Could you check a few things on this model? Use its own coordinates, in mm. A direction names the side the tool comes from. Give positions to 0.01 mm unless a question says otherwise; leave off trailing zeros. Order: outer loops, then holes, each group sorted by start corner. A loop starts at its lowest first (then second) coordinate and runs counter-clockwise, first axis right, second up.
from build123d import *

# Parameters (mm, degrees)
CROQUIS1_W              = 35
CROQUIS1_H              = 28
CROQUIS1_R              = 11
CROQUIS1_R_2            = 1.5
SALIENTE_EXTRUIR1_DEPTH = 10
CROQUIS2_R              = 11
CROQUIS2_R_2            = 9
SALIENTE_EXTRUIR2_DEPTH = 2
REDONDEO1_R             = 14
CHAFL_N1_SIZE           = 2


with BuildPart() as part:
    # Croquis1 → Saliente-Extruir1 (new body)
    with BuildSketch(Plane(origin=(0, 0, 0), x_dir=(0, 1, 0), z_dir=(0, 0, 1))):
        Rectangle(CROQUIS1_W, CROQUIS1_H)
        with Locations(Location((0, 0, 0), (0, 0, 270))):
            Circle(CROQUIS1_R, mode=Mode.SUBTRACT)
        with Locations(Location((-12.5, 8, 0), (0, 0, 270))):
            Circle(CROQUIS1_R_2, mode=Mode.SUBTRACT)
        with Locations(Location((12.5, 8, 0), (0, 0, 90))):
            Circle(CROQUIS1_R_2, mode=Mode.SUBTRACT)
    extrude(amount=SALIENTE_EXTRUIR1_DEPTH)

    # Croquis2 → Saliente-Extruir2 (add)
    with BuildSketch(Plane(origin=(0, 0, 0), x_dir=(0, 1, 0), z_dir=(0, 0, 1))):
        with Locations(Location((0, 0, 0), (0, 0, 270))):
            Circle(CROQUIS2_R)
        with Locations(Location((0, 0, 0), (0, 0, 270))):
            Circle(CROQUIS2_R_2, mode=Mode.SUBTRACT)
    extrude(amount=SALIENTE_EXTRUIR2_DEPTH)

    # Redondeo1
    redondeo1_edges = [part.edges().sort_by_distance(p)[0] for p in [
        (14, 17.5, 5),
        (14, -17.5, 5),
    ]]
    fillet(redondeo1_edges, radius=REDONDEO1_R)

    # Chaflán1
    chafl_n1_edges = [part.edges().sort_by_distance(p)[0] for p in [
        (-14, 0, 0),
    ]]
    chamfer(chafl_n1_edges, length=CHAFL_N1_SIZE)


solid = part.part
Item 1: We'd pull the mould along Y, two halves only. Please class faces 3 (the cylindrical face through (-2.38, -10.74, 5.94)), 4 (the flat face through (-7, -17.5, 5)), 5 (the flat face through (-13, 0, 1)), 6 (the cylindrical face through (10, 13.3, 5.1)): +Y half, -Y half, draft (parallel to the pull), parting line (faces both ways), or undercut.
Findings:
face 3: undercut
face 4: -Y half
face 5: draft
face 6: +Y half
Item 2: Please list where these lines run through material, in increasing order: line 1 along Y through (x, z) = (-8, 6); line 2 along Z through (x, y) = (-9, 3); line 3 along Y through (x, z) = (7.25, 4.75).
Findings:
line 1: y = -17.5 to -14, -11 to -7.55, 7.55 to 11, 14 to 17.5
line 2: z = 0 to 2
line 3: y = -15.48 to -8.27, 8.27 to 15.48
Item 3: Imagine slicing it at D-D on x = -5. List the corners of the cut face in (y, z) for me.
Findings:
outline: (-17.5, 0) - (-7.48, 0) - (-7.48, 2) - (-9.8, 2) - (-9.8, 10) - (-17.5, 10) - close; (7.48, 0) - (17.5, 0) - (17.5, 10) - (9.8, 10) - (9.8, 2) - (7.48, 2) - close
Item 4: Imagine slicing it at C-C on x = -8. List the corners of the cut face in (y, z) for me.
Findings:
outline: (-17.5, 0) - (-14, 0) - (-14, 10) - (-17.5, 10) - close; (-11, 0) - (-4.12, 0) - (-4.12, 2) - (-7.55, 2) - (-7.55, 10) - (-11, 10) - close; (4.12, 0) - (11, 0) - (11, 10) - (7.55, 10) - (7.55, 2) - (4.12, 2) - close; (14, 0) - (17.5, 0) - (17.5, 10) - (14, 10) - close
Item 5: Imagine slicing it at B-B on y = 0. List the corners of the cut face in (x, z) for me.
Findings:
outline: (-14, 2) - (-12, 0) - (-9, 0) - (-9, 2) - (-11, 2) - (-11, 10) - (-14, 10) - close; (9, 0) - (14, 0) - (14, 10) - (11, 10) - (11, 2) - (9, 2) - close
Item 6: For pin 1 (10 mm diameter, centred on x = 5.5, y = -12.5, fed in from -Z); pin 2 (2 mm diameter, centred on x = 5.5, z = 4.5, fed in from +Y), each with a flat end and sliding along its axis, tell me the tip position at first contact or that it passes through.
Findings:
pin 1: stops at z = 0
pin 2: stops at y = 16.76
Item 7: Imagine slicing it at A-A on z = 8.25. List the corners of the cut face in (x, y) for me, then the cut area to 3 significant figures.
Findings:
outline: (-14, -17.5) - (0, -17.5) arc R14 ccw to (14, -3.5) - (14, 3.5) arc R14 ccw to (0, 17.5) - (-14, 17.5) - close; hole circle Ø22 at (0, 0); hole circle Ø3 at (-8, -12.5); hole circle Ø3 at (-8, 12.5)
area: 502 mm2
Item 8: For faces 1 (the flat face through (2, -9, 2)), 2 (the cylindrical face through (9.8, -13.5, 5.1)), which set-ups out of +Z, -Z, +X, -X, +Y, -Y let a thin tool reach every point of the face, with its end or its side?
Findings:
face 1: +Z
face 2: +Z, -Z, +X, -Y
